```python
from build123d import *

# Parameters (mm, degrees)
SKETCH1_R           = 20
BOSS_EXTRUDE1_DEPTH = 80
BOSS_EXTRUDE2_DEPTH = 110


with BuildPart() as part:
    # Sketch1 → Boss-Extrude1 (new, symmetric)
    with BuildSketch(Plane(origin=(0, 0, 0), x_dir=(1, 0, 0), z_dir=(0, 1, 0))):
        with Locations(Location((0, 0, 0), (0, 0, 270))):
            Circle(SKETCH1_R)
    extrude(amount=BOSS_EXTRUDE1_DEPTH, both=True)

    # Sketch2 → Boss-Extrude2 (add)
    with BuildSketch(Plane(origin=(0, 80, 0), x_dir=(1, 0, 0), z_dir=(0, 1, 0))):
        with BuildLine():
            ThreePointArc((-19.364916731, -5), (-20, 0), (-19.364916731, 5))
            Line((-19.364916731, 5), (-24.364916731, 5))
            Line((-24.364916731, 5), (-24.364916731, -5))
            Line((-24.364916731, -5), (-19.364916731, -5))
        make_face()
    extrude(amount=-BOSS_EXTRUDE2_DEPTH)


solid = part.part
```
CAD build for the part. Positions are in the model's coordinates, mm. A direction names the side the tool comes from. Coordinates: 2 decimals unless noted, no trailing zeros. Order: outer loops, then holes, each group sorted by start corner. A loop starts at its lowest first (then second) coordinate and runs counter-clockwise, first axis right, second up.
(1) Saw through at D-D, the plane y = 22.5. Write the cut outline in (x, z).
Solution:
outline: (-24.36, -5) - (-19.36, -5) arc R20 ccw (long way) to (-19.36, 5) - (-24.36, 5) - close
(2) Pin check, flat tips, straight feed: pin 1 Ø2 at (x, y) = (-2, 33) entering from -Z (3 decimals); pin 2 Ø12 at (x, z) = (14.5, 14.5) entering from +Y; pin 3 Ø1.5 at (x, y) = (-22.5, 24) entering from -Z; pin 4 Ø5 at (x, y) = (9.5, 18.5) entering from +Z (3 decimals). Stop position of each tip, or through.
Solution:
pin 1: stops at z = -19.975
pin 2: stops at y = 80
pin 3: stops at z = -5
pin 4: stops at z = 18.735
(3) Saw through at C-C, the plane x = -5. Write the cut outline in (y, z), and give its area (3 significant figures).
Solution:
outline: (-80, -19.36) - (80, -19.36) - (80, 19.36) - (-80, 19.36) - close
area: 6,200 mm2
(4) Drill centre lines: L1, parallel to X at y = -34.5, z = -1; L2, parallel to Z at x = 11, y = -60.5. Where is each one in solid material? Low to high.
Solution:
L1: x = -19.97 to 19.97
L2: z = -16.7 to 16.7
(5) Saw through at B-B, the plane y = -52. Write the cut outline in (x, z), and give its area (3 significant figures).
Solution:
outline: circle Ø40 at (0, 0)
area: 1,260 mm2
(6) Saw through at A-A, the plane z = 0. Write the cut outline in (x, y), and give its area (3 significant figures).
Solution:
outline: (-24.36, -30) - (-20, -30) - (-20, -80) - (20, -80) - (20, 80) - (-24.36, 80) - close
area: 6,880 mm2
(7) Which spindle directions (+Z, -Z, +X, -X, +Y, -Y) get a long thin tool onto all of the face, cutting with end or side? Do faces 1 (the face through (-22, 26, -5)), 2 (the face through (0, -80, 0)), 3 (the face through (-22, 26, 5)). Say none if no direction does.
Solution:
face 1: -Z, -X, +Y, -Y
face 2: +Z, -Z, +X, -X, -Y
face 3: +Z, -X, +Y, -Y
